from build123d import *

# Parameters (mm, degrees)
BOSS_EXTRUDE1_DEPTH = 3.5
FILLET1_R           = 0.6
CUT_EXTRUDE1_DEPTH  = 4
CUT_EXTRUDE2_DEPTH  = 10


with BuildPart() as part:
    # Sketch1 → Boss-Extrude1 (new body)
    with BuildSketch(Plane(origin=(0, 0, 0), x_dir=(1, 0, 0), z_dir=(0, 1, 0))):
        Polygon((0, 0), (0, 1.9), (-0.6, 1.9), (-0.6, -0.6), (5.7, -0.6), (5.7, 3), (5.1, 3), (5.1, 0), align=None)
    extrude(amount=BOSS_EXTRUDE1_DEPTH)

    # Fillet1
    fillet1_edges = [part.edges().sort_by_distance(p)[0] for p in [
        (5.1, 1.75, 0),
        (5.7, 1.75, 0.6),
        (-0.6, 1.75, 0.6),
        (0, 1.75, 0),
    ]]
    fillet(fillet1_edges, radius=FILLET1_R)

    # Sketch2 → Cut-Extrude1 (cut)
    with BuildSketch(Plane(origin=(5.7, 0, 0), x_dir=(0, 0, -1), z_dir=(1, 0, 0))):
        with BuildLine():
            Line((2, 3), (3, 3))
            Line((3, 3), (3, 0.5))
            Line((3, 0.5), (2, 0.5))
            ThreePointArc((2, 0.5), (0.75, 1.75), (2, 3))
        make_face()
    extrude(amount=-CUT_EXTRUDE1_DEPTH, mode=Mode.SUBTRACT)

    # Sketch3 → Cut-Extrude2 (cut)
    with BuildSketch(Plane.ZY.offset(0.6)):
        with BuildLine():
            Line((-1.9, 0.75), (-1.9, 2.75))
            ThreePointArc((-1.9, 2.75), (-0.9, 1.75), (-1.9, 0.75))
        make_face()
    extrude(amount=-CUT_EXTRUDE2_DEPTH, mode=Mode.SUBTRACT)


solid = part.part
Input: part model. Units: mm. Frame: model coordinates. A direction names the side the tool comes from. Give positions to 0.01 mm unless a question says otherwise; leave off trailing zeros. Loops run counter-clockwise (first coordinate to the right, second up) from the corner with the lowest first, then second, coordinate; pieces in that order, holes last. Notation, with made-up numbers: (86, 46) -> (104, 46) arc R22 ccw to (104, 74) -> close; hole circle Ø6 at (27.5, 29). An arc over 180 degrees is marked (long way). Answer as a JSON object with one key per item and string values. Group by question number.
Item 1: Cut plane B-B, the plane z = -1.8. Return the cut outline in (x, y), and give its area (3 significant figures).
Item 2: Pull-direction query (X, two-part tool) for faces 4 (the flat face through (2.8, 3.5, 0.3)), 5 (the flat face through (-0.6, 1.73, -0.75)), 6 (the flat face through (0, 1, -1)); classes: released by +X, released by -X, zero draft, split by the parting line, or undercut.
Item 3: Reachability of faces 1 (the flat face through (3, 2, 0)), 2 (the cylindrical face through (5.4, 1.72, -0.75)), 3 (the flat face through (3, 2, 0.6)) from +Z, -Z, +X, -X, +Y, -Y: full face, straight path, thin tool, end or side. Return the list, or none.
Item 4: Line query: probe 1 along X at (y, z) = (3.05, -1.3); probe 2 along Y at (x, z) = (5.5, -2.75); probe 3 along Z at (x, y) = (3.25, 0.8). Output: solid intervals per line, ascending.
Item 5: Cut plane A-A, the plane y = 1.8. Return the cut outline in (x, z), and give its area (3 significant figures).
Item 6: Pin query (flat end, axial travel): P1, Ø1.2, axis at y = 2, z = -1.5, coming from the -X side; P2, Ø0.7, axis at x = -0.5, y = 0, coming from the -Z side. Return the tip coordinate at first contact, or that it passes through.
Item 7: Cut plane D-D, the plane z = -0.3. Return the cut outline in (x, y).
Item 8: Cut plane C-C, the plane x = 2.25. Return the cut outline in (y, z).
Checks:
{
 "1": {"outline": "(-0.6, 0) -> (0, 0) -> (0, 0.76) -> (-0.6, 0.76) -> close; (-0.6, 2.74) -> (0, 2.74) -> (0, 3.5) -> (-0.6, 3.5) -> close; (5.1, 0) -> (5.7, 0) -> (5.7, 0.52) -> (5.1, 0.52) -> close; (5.1, 2.98) -> (5.7, 2.98) -> (5.7, 3.5) -> (5.1, 3.5) -> close", "area": "1.53 mm²"},
 "2": {"face 4": "zero draft", "face 5": "released by -X", "face 6": "undercut"},
 "3": {"face 1": "-Z, +Y, -Y", "face 2": "-Z, +X", "face 3": "+Z, +X, -X, +Y, -Y"},
 "4": {"probe 1": "x = -0.6 to 0, 5.1 to 5.7", "probe 2": "y = 0 to 0.5, 3 to 3.5", "probe 3": "z = 0 to 0.6"},
 "5": {"outline": "(-0.6, -0.9) -> (0, -0.9) -> (0, -0.6) arc R0.6 cw to (0.6, 0) -> (4.5, 0) arc R0.6 cw to (5.1, -0.6) -> (5.1, -0.75) -> (5.7, -0.75) -> (5.7, 0) arc R0.6 ccw to (5.1, 0.6) -> (0, 0.6) arc R0.6 ccw to (-0.6, 0) -> close", "area": "4.77 mm²"},
 "6": {"P1": "stops at x = -0.6", "P2": "stops at z = -1.9"},
 "7": {"outline": "(-0.6, 0) -> (0.08, 0) -> (0.08, 3.5) -> (-0.6, 3.5) -> close; (5.02, 0) -> (5.7, 0) -> (5.7, 3.5) -> (5.02, 3.5) -> close"},
 "8": {"outline": "(0, 0) -> (3.5, 0) -> (3.5, 0.6) -> (0, 0.6) -> close"}
}
